Could you check a few things on this drawing? It's one solid part, dimensions in mm from its lowest x, y, z. Round coordinates to 2 decimals unless told otherwise and drop trailing zeros. Write each loop counter-clockwise with the first axis right and the second up, starting at its lowest first coordinate (ties: lowest second). Pieces come first, ordered by that corner, then holes. Notation, with made-up numbers: (-35, -25) - (-19, -25) arc R21 ccw to (-19, -16) - close; hole circle Ø3 at (57, 65.25). An arc over 180 degrees is marked (long way). Write item = value, one per line. Start each with the question number.
Item 1: If we section it at B-B (x = 92): Please give me the cut outline in (y, z), and give its area (3 significant figures).
Item 2: If we section it at A-A (z = 1): Please give me the cut outline in (x, y), and give its area (3 significant figures).
Item 3: For P1, Ø1.5, axis at y = 41, z = 2, coming from the +X side; P2, Ø3, axis at x = 146, z = 3, coming from the +Y side; P3, Ø1.2, axis at x = 1.5, z = 3.5, coming from the -Y side, each with a flat end and sliding along its axis, tell me the tip position at first contact or that it passes through.
Item 4: If I drill on line 1 along X through (y, z) = (36, 1.25); line 2 along X through (y, z) = (6.5, 0.55); line 3 along Y through (x, z) = (111.5, 2.25), over which ranges is the centre line in solid material (lowest first)? Write a range as [from, to].
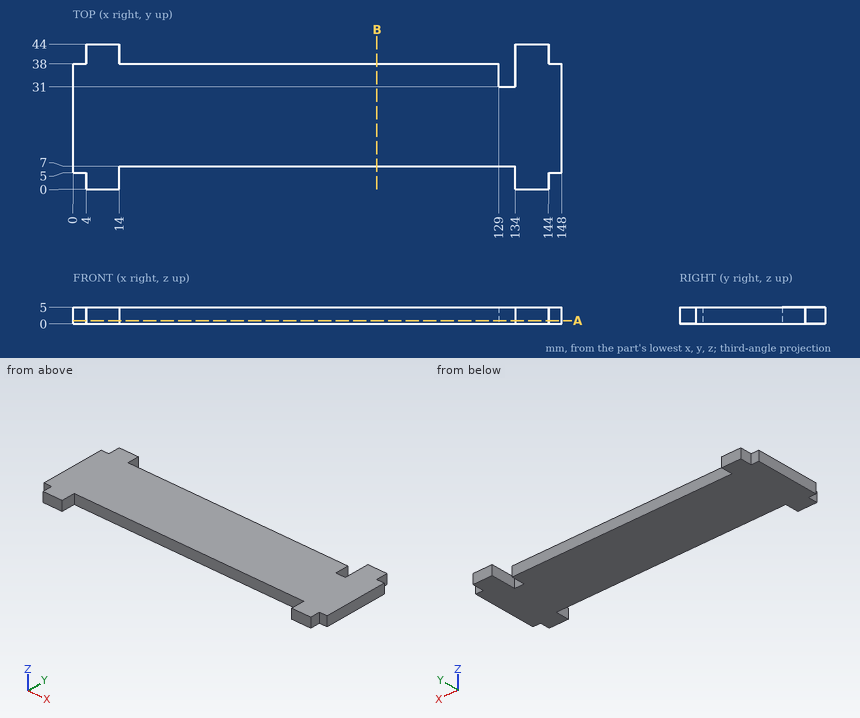
Reply:
q1.outline = (7, 0) - (38, 0) - (38, 5) - (7, 5) - close
q1.area = 155 mm2
q2.outline = (0, 5) - (4, 5) - (4, 0) - (14, 0) - (14, 7) - (134, 7) - (134, 0) - (144, 0) - (144, 5) - (148, 5) - (148, 38) - (144, 38) - (144, 44) - (134, 44) - (134, 31) - (129, 31) - (129, 38) - (14, 38) - (14, 44) - (4, 44) - (4, 38) - (0, 38) - close
q2.area = 4,830 mm2
q3.P1 = 144
q3.P2 = 38
q3.P3 = 5
q4.line_1 = [0, 129], [134, 148]
q4.line_2 = [0, 14], [134, 148]
q4.line_3 = [7, 38]
